```python
from build123d import *

# Parameters (mm, degrees)
BOSS_EXTRUDE3_DEPTH = 5
SKETCH4_R           = 1.5
CUT_EXTRUDE1_DEPTH  = 70
SKETCH5_R           = 2.1
SKETCH5_W           = 41
SKETCH5_H           = 21
CUT_EXTRUDE2_DEPTH  = 10
SKETCH6_W           = 5
SKETCH6_H           = 52
BOSS_EXTRUDE4_DEPTH = 36.8
BOSS_EXTRUDE5_DEPTH = 5
SKETCH8_R           = 4.1
BOSS_EXTRUDE6_DEPTH = 40
SKETCH10_R          = 4.1
CUT_EXTRUDE5_DEPTH  = 25
FILLET2_R           = 4


with BuildPart() as part:
    # Sketch3 → Boss-Extrude3 (new body)
    with BuildSketch(Plane(origin=(0, 0, 0), x_dir=(0, 0, -1), z_dir=(1, 0, 0))):
        with BuildLine():
            Line((-75.75, 26), (75.75, 26))
            ThreePointArc((75.75, 26), (101.75, 0), (75.75, -26))
            Line((75.75, -26), (-75.75, -26))
            ThreePointArc((-75.75, -26), (-101.75, 0), (-75.75, 26))
        make_face()
    extrude(amount=BOSS_EXTRUDE3_DEPTH)

    # Sketch4 → Cut-Extrude1 (cut)
    with BuildSketch(Plane.ZY):
        with Locations((-75.75, 0)):
            Circle(SKETCH4_R)
        with Locations((-75.75, 7)):
            Circle(SKETCH4_R)
        with Locations((-68.75, 0)):
            Circle(SKETCH4_R)
        with Locations((-75.75, -7)):
            Circle(SKETCH4_R)
        with Locations((-82.75, 0)):
            Circle(SKETCH4_R)
    extrude(amount=-CUT_EXTRUDE1_DEPTH, mode=Mode.SUBTRACT)

    # Sketch5 → Cut-Extrude2 (cut)
    with BuildSketch(Plane.ZY):
        with Locations((89.6, 5)):
            Circle(SKETCH5_R)
        with Locations(Location((89.6, -5, 0), (0, 0, 180))):
            Circle(SKETCH5_R)
        with Locations((38.6, -5)):
            Circle(SKETCH5_R)
        with Locations(Location((38.6, 5, 0), (0, 0, 180))):
            Circle(SKETCH5_R)
        with Locations((64.1, 0)):
            Rectangle(SKETCH5_W, SKETCH5_H)
    extrude(amount=-CUT_EXTRUDE2_DEPTH, mode=Mode.SUBTRACT)

    # Sketch6 → Boss-Extrude4 (add)
    with BuildSketch(Plane(origin=(5, 0, 0), x_dir=(0, 0, -1), z_dir=(1, 0, 0))):
        with Locations((27.431638641, 0)):
            Rectangle(SKETCH6_W, SKETCH6_H)
        with Locations((-2.568361359, 0)):
            Rectangle(SKETCH6_W, SKETCH6_H)
    extrude(amount=BOSS_EXTRUDE4_DEPTH)

    # Sketch7 → Boss-Extrude5 (add)
    with BuildSketch(Plane(origin=(41.8, 0, 0), x_dir=(0, 0, -1), z_dir=(1, 0, 0))):
        with BuildLine():
            Line((-75.75, 26), (75.75, 26))
            ThreePointArc((75.75, 26), (101.75, 0), (75.75, -26))
            Line((75.75, -26), (-75.75, -26))
            ThreePointArc((-75.75, -26), (-101.75, 0), (-75.75, 26))
        make_face()
    extrude(amount=BOSS_EXTRUDE5_DEPTH)

    # Sketch8 → Boss-Extrude6 (add)
    with BuildSketch(Plane.ZY.offset(-41.8)):
        with Locations((-75.75, 0)):
            Circle(SKETCH8_R)
    extrude(amount=-BOSS_EXTRUDE6_DEPTH)

    # Sketch10 → Cut-Extrude5 (cut)
    with BuildSketch(Plane(origin=(46.8, 0, 0), x_dir=(0, 0, -1), z_dir=(1, 0, 0))):
        with Locations((-74.25, 0)):
            Circle(SKETCH10_R)
    extrude(amount=-CUT_EXTRUDE5_DEPTH, mode=Mode.SUBTRACT)

    # Fillet2
    fillet2_edges = [part.edges().sort_by_distance(p)[0] for p in [
        (41.8, 0, 5.068361359),
        (41.8, 0, 0.068361359),
        (5, 0, -29.931638641),
        (5, 0, -24.931638641),
        (41.8, 0, -29.931638641),
        (41.8, 0, -24.931638641),
        (5, 0, 5.068361359),
        (5, 0, 0.068361359),
    ]]
    fillet(fillet2_edges, radius=FILLET2_R)


solid = part.part
```
Check sheet for the modelled part. Datum: model origin and axes. Units: mm. A direction names the side the tool comes from. Round coordinates to 2 decimals unless told otherwise and drop trailing zeros. Loops run counter-clockwise (first coordinate to the right, second up) from the corner with the lowest first, then second, coordinate; pieces in that order, holes last. Notation, with made-up numbers: (6.5, 80.5) -> (11.5, 80.5) arc R33 ccw to (11.5, 117.5) -> close; hole circle Ø10 at (-19.5, 76). An arc over 180 degrees is marked (long way). Answer in a Markdown table with one row per item.
Q1. Sectioned sample at B-B on x = 21.5. Enter the section's corners in (y, z), then the cut area to 3 significant figures.
Data:
| item | result |
|---|---|
| outline | (-26, -29.93) -> (26, -29.93) -> (26, -24.93) -> (-26, -24.93) -> close; (-26, 0.07) -> (26, 0.07) -> (26, 5.07) -> (-26, 5.07) -> close |
| area | 520 mm^2 |
Q2. Set-up check for faces 5 (the face through (2.46, 6.77, 90.73)), 6 (the face through (6.14, 0.36, 6.27)), 7 (the face through (6.203, 0.364, -1.072)), 8 (the face through (2.465, 0.572, -101.744)): record each of +Z, -Z, +X, -X, +Y, -Y from which the full face is reachable in a straight line by a thin tool's end or side.
Data:
| item | result |
|---|---|
| face 5 | -X |
| face 6 | +Z, +Y, -Y |
| face 7 | +Y, -Y |
| face 8 | -Z, +X, -X |
Q3. Sectioned sample at C-C on z = 38.6. Enter the section's corners in (x, y).
Data:
| item | result |
|---|---|
| outline | (0, -26) -> (5, -26) -> (5, -7.1) -> (0, -7.1) -> close; (0, -2.9) -> (5, -2.9) -> (5, 2.9) -> (0, 2.9) -> close; (0, 7.1) -> (5, 7.1) -> (5, 26) -> (0, 26) -> close; (41.8, -26) -> (46.8, -26) -> (46.8, 26) -> (41.8, 26) -> close |
Q4. Sectioned sample at A-A on z = -41. Enter the section's corners in (x, y), then the cut area to 3 significant figures.
Data:
| item | result |
|---|---|
| outline | (0, -26) -> (5, -26) -> (5, 26) -> (0, 26) -> close; (41.8, -26) -> (46.8, -26) -> (46.8, 26) -> (41.8, 26) -> close |
| area | 520 mm^2 |
Q5. Release check for a two-part mould opening along X. For faces 1 (the face through (5, 0, -61)), 2 (the face through (44.265, 0.572, -101.744)), 3 (the face through (5, 12, 55)), 4 (the face through (46.8, 0, -1)) record: released by +X, released by -X, zero draft, split by the parting line, or undercut.
Data:
| item | result |
|---|---|
| face 1 | undercut |
| face 2 | zero draft |
| face 3 | undercut |
| face 4 | released by +X |
Q6. Thickness scan on L1, parallel to Y at x = 1.8, z = -75.75; L2, parallel to Z at x = 33.5, y = 11; L3, parallel to X at y = -6, z = -79. Record the ranges inside material, lowest first.
Data:
| item | result |
|---|---|
| L1 | y = -26 to -8.5, -5.5 to -1.5, 1.5 to 5.5, 8.5 to 26 |
| L2 | z = -29.93 to -24.93, 0.07 to 5.07 |
| L3 | x = 0 to 5, 41.8 to 46.8 |
Q7. Sectioned sample at D-D on y = -14. Enter the section's corners in (x, z), then the cut area to 3 significant figures.
Data:
| item | result |
|---|---|
| outline | (0, -97.66) -> (5, -97.66) -> (5, -33.93) arc R4 cw to (9, -29.93) -> (37.8, -29.93) arc R4 cw to (41.8, -33.93) -> (41.8, -97.66) -> (46.8, -97.66) -> (46.8, 97.66) -> (41.8, 97.66) -> (41.8, 9.07) arc R4 cw to (37.8, 5.07) -> (9, 5.07) arc R4 cw to (5, 9.07) -> (5, 97.66) -> (0, 97.66) -> close; hole (5, -20.93) arc R4 ccw to (9, -24.93) -> (37.8, -24.93) arc R4 ccw to (41.8, -20.93) -> (41.8, -3.93) arc R4 ccw to (37.8, 0.07) -> (9, 0.07) arc R4 ccw to (5, -3.93) -> close |
| area | 2,350 mm^2 |
Q8. Go/stop test with flat-tipped pins: P1, Ø1.5, axis at y = -5.5, z = -53, coming from the +X side; P2, Ø2.5, axis at y = -5, z = 38.6, coming from the -X side; P3, Ø6, axis at x = 36.5, y = -1, coming from the -Z side. Record where each tip stops, or that it passes through.
Data:
| item | result |
|---|---|
| P1 | stops at x = 46.8 |
| P2 | stops at x = 41.8 |
| P3 | stops at z = -30.31 |
